Here's how the part is built. I have some questions about the finished solid (model axes, mm). A direction names the side the tool comes from. Give positions to 0.01 mm unless a question says otherwise; leave off trailing zeros. Loops run counter-clockwise (first coordinate to the right, second up) from the corner with the lowest first, then second, coordinate; pieces in that order, holes last. Notation, with made-up numbers: (72.25, -40) -> (115.25, -40) arc R14 ccw to (115.25, -22) -> close; hole circle Ø5 at (-6.5, 89.5). An arc over 180 degrees is marked (long way). Answer in a Markdown table with one row per item. Add a question column.
Item 1: If we section it at B-B (y = -7.75): Write out the boundary of the cut face in (x, z) (3 decimals).
Item 2: Which directions (+Z, -Z, +X, -X, +Y, -Y) give clear straight access to the entire face, cutting with the end or side of a thin tool? Please do faces 1 (the face through (-1.07, -5.73, 1.05)), 2 (the face through (-0.5, -6, -2)), 3 (the face through (2, -6, 0.5)), 4 (the face through (0.5, -6, -2)).
Item 3: If we section it at A-A (y = -5.5): Write out the boundary of the cut face in (x, z) (3 decimals), then the cut area to 3 significant figures.
Item 4: If I drill on line 1 (Z direction, x = 0, y = -7.05) (3 decimals); line 2 (Y direction, x = 0.25, z = -1), over which ranges is the centre line in solid material (lowest first)?
Item 5: If we section it at D-D (y = -13): Write out the boundary of the cut face in (x, z).
Item 6: For P1, Ø0.9, axis at x = -2, y = -6, coming from the -Z side; P2, Ø0.9, axis at y = -5.5, z = 2, coming from the -X side; P3, Ø0.9, axis at y = -7, z = 1.5, coming from the +X side, each with a flat end and sliding along its axis, tell me the tip position at first contact or that it passes through.
Item 7: We'd pull the mould along Z, two halves only. Please class faces 5 (the face through (1.34, -7.63, 1.32)), 6 (the face through (1, -8, 0)), 7 (the face through (0.5, -6, 2)): released by +Z, released by -Z, zero draft, split by the parting line, or undercut.
Item 8: If we section it at C-C (y = -11.25): Write out the boundary of the cut face in (x, z).
Autodesk Inventor part; units mm, degrees
ref_plane "YZ Plane" through (0, 0, 0) normal (1, 0, 0) x (0, 1, 0)
ref_plane "XZ Plane" through (0, 0, 0) normal (0, 1, 0) x (-1, 0, 0)
ref_plane "XY Plane" through (0, 0, 0) normal (0, 0, 1) x (1, 0, 0)
sketch "Sketch1" plane through (0, 0, 0) normal (0, 1, 0) x (-1, 0, 0)
  circle A0 centre (0, 0) radius 0.525
  circle A1 centre (0, 0) radius 0.625
  dimension "d0" = 1.25
  dimension "d1" = 0.1
extrude "Extrusion1" add sketch "Sketch1" along normal blind 25
sketch "Sketch2" plane through (0, 0, 0) normal (1, 0, 0) x (0, 1, 0)
  line L0 (25, -0.625) -> (25, 0.625) construction
  line L1 (25, 0.625) -> (23.5, -0.625)
  line L2 (25, 0.625) -> (25, -0.625)
  line L3 (25, -0.625) -> (23.5, -0.625)
  point P0 (0, 0)
  dimension "d4" = 1.5
extrude "Extrusion2" cut sketch "Sketch2" along normal through all both and the other way through all
sketch "Sketch3" plane through (0, 0, 0) normal (0, -1, 0) x (1, 0, 0)
  circle A0 centre (0, 0) radius 1.5
  circle A1 centre (0, 0) radius 0.625
  circle A2 centre (0, 0) radius 0.625 construction
  dimension "d7" = 3
extrude "Extrusion3" add sketch "Sketch3" along normal blind 1 separate body
sketch "Sketch4" plane through (0, -1, 0) normal (0, -1, 0) x (1, 0, 0)
  line L0 (0.5, -1.4142) -> (0.5, -2.25)
  line L1 (0.5, -2.25) -> (-0.5, -2.25)
  line L2 (-0.5, -2.25) -> (-0.5, -1.4142)
  arc A0 (-0.5, -1.4142) -> (0.5, -1.4142) centre (0, 0) ccw
  circle A1 centre (0, 0) radius 1.5
  line L3 (1.4142, 0.5) -> (2.25, 0.5)
  line L4 (2.25, 0.5) -> (2.25, -0.5)
  line L5 (2.25, -0.5) -> (1.4142, -0.5)
  arc A2 (1.4142, -0.5) -> (1.4142, 0.5) centre (0, 0) ccw
  line L6 (-0.5, 1.4142) -> (-0.5, 2.25)
  line L7 (-0.5, 2.25) -> (0.5, 2.25)
  line L8 (0.5, 2.25) -> (0.5, 1.4142)
  arc A3 (0.5, 1.4142) -> (-0.5, 1.4142) centre (0, 0) ccw
  line L9 (-1.4142, -0.5) -> (-2.25, -0.5)
  line L10 (-2.25, -0.5) -> (-2.25, 0.5)
  line L11 (-2.25, 0.5) -> (-1.4142, 0.5)
  arc A4 (-1.4142, 0.5) -> (-1.4142, -0.5) centre (0, 0) ccw
  circle A5 centre (0, 0) radius 1.5 construction
  circle A6 centre (0, 0) radius 1.5 construction
  circle A7 centre (0, 0) radius 1.5
  circle A8 centre (0, 0) radius 1.3
  dimension "d20" = 2.25
  dimension "d21" = 1
  dimension "d24" = 360
  dimension "d26" = 0.2
extrude "Extrusion4" add sketch "Sketch4" along normal blind 7 bodies 2
sketch "Sketch5" plane through (0, 0, 0) normal (0, 0, 1) x (1, 0, 0)
  line L0 (1.3, -8) -> (-1.3, -8) construction
  line L1 (-1.3, -8) -> (-2.1, -18)
  line L2 (-2.1, -18) -> (-3.25, -18)
  line L3 (-3.25, -18) -> (-3.25, -17)
  line L4 (-3.25, -17) -> (-3, -17)
  line L5 (-2.25, -8) -> (-1.4142, -8) construction
  line L6 (-3, -17) -> (-2.25, -8)
  line L7 (-2.25, -8) -> (-1.3, -8)
  line L8 (0, -26.6) -> (0, 33.6)
  point P0 (0, 0)
  dimension "d27" = 2.1
  dimension "d28" = 3.25
  dimension "d29" = 3
  dimension "d30" = 9
  dimension "d31" = 1
revolve "Revolution1" add sketch "Sketch5" angle 360 about axis through (0, -10, 0) along (0, 1, 0) bodies 2
chamfer "Chamfer1" distance 0.25 angle 45 4 edges at (2.25, -1, 0) (0, -1, -2.25) (-2.25, -1, 0) (0, -1, 2.25)
chamfer "Chamfer2" distance 0.75 angle 45 4 edges at (1.0607, -8, 1.0607) (1.0607, -8, -1.0607) (-1.0607, -8, -1.0607) (-1.0607, -8, 1.0607)
sketch "Sketch7" plane through (0, 0, 0) normal (0, 1, 0) x (1, 0, 0)
  circle A0 centre (0, 0) radius 0.625
  circle A1 centre (0, 0) radius 2.3049
  point P0 (0.5, 2.25)
extrude "Extrusion6" cut sketch "Sketch7" along normal blind 30 and the other way blind 4.25 contours A0 | A1 bodies 2 1
sketch "Sketch8" plane through (0, -4.25, 0) normal (0, 1, 0) x (1, 0, 0)
  circle A0 centre (0, 0) radius 0.625
  circle A1 centre (0, 0) radius 1.3
  dimension "d49" = 1.25
extrude "Extrusion7" add sketch "Sketch8" against normal blind 3.75 bodies 2
properties part number "CH_01_0030_needle_1"
Recorded:
| question | item | result |
|---|---|---|
| 1 | outline | (-2.25, -0.5) -> (-1.936, -0.5) arc R2 ccw to (-0.5, -1.936) -> (-0.5, -2.25) -> (0.5, -2.25) -> (0.5, -1.936) arc R2 ccw to (1.936, -0.5) -> (2.25, -0.5) -> (2.25, 0.5) -> (1.936, 0.5) arc R2 ccw to (0.5, 1.936) -> (0.5, 2.25) -> (-0.5, 2.25) -> (-0.5, 1.936) arc R2 ccw to (-1.936, 0.5) -> (-2.25, 0.5) -> close; hole circle Ø1.25 at (0, 0) |
| 2 | face 1 | +Z, -X, +Y |
| 2 | face 2 | -Z, -X, +Y |
| 2 | face 3 | +Z, +X, +Y |
| 2 | face 4 | -Z, +X, +Y |
| 3 | outline | (-2.25, -0.5) -> (-1.414, -0.5) arc R1.5 ccw to (-0.5, -1.414) -> (-0.5, -2.25) -> (0.5, -2.25) -> (0.5, -1.414) arc R1.5 ccw to (1.414, -0.5) -> (2.25, -0.5) -> (2.25, 0.5) -> (1.414, 0.5) arc R1.5 ccw to (0.5, 1.414) -> (0.5, 2.25) -> (-0.5, 2.25) -> (-0.5, 1.414) arc R1.5 ccw to (-1.414, 0.5) -> (-2.25, 0.5) -> close; hole circle Ø1.25 at (0, 0) |
| 3 | area | 8.95 mm^2 |
| 4 | line 1 | z = -2.25 to -0.625, 0.625 to 2.25 |
| 4 | line 2 | y = -8 to -4.25 |
| 5 | outline | circle Ø5.33 at (0, 0); hole circle Ø3.4 at (0, 0) |
| 6 | P1 | stops at z = -0.5 |
| 6 | P2 | stops at x = -0.5 |
| 6 | P3 | stops at x = 1.07 |
| 7 | face 5 | released by +Z |
| 7 | face 6 | undercut |
| 7 | face 7 | zero draft |
| 8 | outline | circle Ø5.04 at (0, 0); hole circle Ø3.12 at (0, 0) |
